from build123d import *

# Parameters (mm, degrees)
CROQUIS1_R              = 100
SALIENTE_EXTRUIR1_DEPTH = 3
CROQUIS3_R              = 110
CORTAR_EXTRUIR1_DEPTH   = 3
REDONDEO1_R             = 10
CROQUIS4_R              = 1.5
CROQUIS4_R_2            = 12.5
CORTAR_EXTRUIR2_DEPTH   = 142.453172607
CROQUIS5_R              = 1.5
CORTAR_EXTRUIR3_DEPTH   = 142.453172607
CROQUIS7_R              = 2
CORTAR_EXTRUIR5_DEPTH   = 10


with BuildPart() as part:
    # Croquis1 → Saliente-Extruir1 (new body)
    with BuildSketch(Plane.XY):
        Circle(CROQUIS1_R)
    extrude(amount=SALIENTE_EXTRUIR1_DEPTH)

    # Croquis3 → Cortar-Extruir1 (cut)
    with BuildSketch(Plane.XY.offset(3)):
        with Locations((190, 0)):
            Circle(CROQUIS3_R)
    extrude(amount=-CORTAR_EXTRUIR1_DEPTH, mode=Mode.SUBTRACT)

    # Redondeo1
    redondeo1_edges = [part.edges().sort_by_distance(p)[0] for p in [
        (89.473684211, -44.659375654, 1.5),
        (89.473684211, 44.659375654, 1.5),
    ]]
    fillet(redondeo1_edges, radius=REDONDEO1_R)

    # Croquis4 → Cortar-Extruir2 (cut, through all)
    with BuildSketch(Plane.XY.offset(3)):
        with Locations((-65.01846853, -38.219121523)):
            Circle(CROQUIS4_R)
        with Locations((-49.462119344, -22.662772337)):
            Circle(CROQUIS4_R)
        with Locations((-22.662772337, -49.462119344)):
            Circle(CROQUIS4_R)
        with Locations((-38.219121523, -65.01846853)):
            Circle(CROQUIS4_R)
        with Locations((-22.662772337, 49.462119344)):
            Circle(CROQUIS4_R)
        with Locations((-38.219121523, 65.01846853)):
            Circle(CROQUIS4_R)
        with Locations((-49.462119344, 22.662772337)):
            Circle(CROQUIS4_R)
        with Locations((-65.01846853, 38.219121523)):
            Circle(CROQUIS4_R)
        with Locations((49.462119344, 22.662772337)):
            Circle(CROQUIS4_R)
        with Locations((65.01846853, 38.219121523)):
            Circle(CROQUIS4_R)
        with Locations((22.662772337, 49.462119344)):
            Circle(CROQUIS4_R)
        with Locations((38.219121523, 65.01846853)):
            Circle(CROQUIS4_R)
        with Locations((22.662772337, -49.462119344)):
            Circle(CROQUIS4_R)
        with Locations((38.219121523, -65.01846853)):
            Circle(CROQUIS4_R)
        with Locations((49.462119344, -22.662772337)):
            Circle(CROQUIS4_R)
        with Locations((65.01846853, -38.219121523)):
            Circle(CROQUIS4_R)
        Circle(CROQUIS4_R_2)
        Polygon((-58.336309448, -83.085046789), (-83.085046789, -58.336309448), (-66.821590822, -42.072853481), (-42.072853481, -66.821590822), align=None)
        Polygon((-66.821590822, 42.072853481), (-42.072853481, 66.821590822), (-58.336309448, 83.085046789), (-83.085046789, 58.336309448), align=None)
        Polygon((42.072853481, 66.821590822), (66.821590822, 42.072853481), (83.085046789, 58.336309448), (58.336309448, 83.085046789), align=None)
        Polygon((66.821590822, -42.072853481), (42.072853481, -66.821590822), (58.336309448, -83.085046789), (83.085046789, -58.336309448), align=None)
    extrude(amount=-CORTAR_EXTRUIR2_DEPTH, mode=Mode.SUBTRACT)

    # Croquis5 → Cortar-Extruir3 (cut, through all)
    with BuildSketch(Plane(origin=(0, 0, 0), x_dir=(-1, 0, 0), z_dir=(0, 0, -1))):
        with Locations((11.5, -90)):
            Circle(CROQUIS5_R)
        with Locations((-11.5, -90)):
            Circle(CROQUIS5_R)
        with Locations((-11.5, -50)):
            Circle(CROQUIS5_R)
        with Locations((11.5, -50)):
            Circle(CROQUIS5_R)
        with Locations((-11.5, 90)):
            Circle(CROQUIS5_R)
        with Locations((11.5, 90)):
            Circle(CROQUIS5_R)
        with Locations((11.5, 50)):
            Circle(CROQUIS5_R)
        with Locations((-11.5, 50)):
            Circle(CROQUIS5_R)
    extrude(amount=-CORTAR_EXTRUIR3_DEPTH, mode=Mode.SUBTRACT)

    # Croquis7 → Cortar-Extruir5 (cut)
    with BuildSketch(Plane(origin=(0, 0, 0), x_dir=(-1, 0, 0), z_dir=(0, 0, -1))):
        with Locations((-27.065, -80.785)):
            Circle(CROQUIS7_R)
        with Locations((27.065, -80.785)):
            Circle(CROQUIS7_R)
        with Locations(Location((27.065, 80.785, 0), (0, 0, 180))):
            Circle(CROQUIS7_R)
        with Locations(Location((-27.065, 80.785, 0), (0, 0, 180))):
            Circle(CROQUIS7_R)
    extrude(amount=-CORTAR_EXTRUIR5_DEPTH, mode=Mode.SUBTRACT)


solid = part.part
Geometry: final body of the model. Coordinates: model frame, mm. A direction names the side the tool comes from. Round coordinates to 2 decimals unless told otherwise and drop trailing zeros. Loops run counter-clockwise (first coordinate to the right, second up) from the corner with the lowest first, then second, coordinate; pieces in that order, holes last. Notation, with made-up numbers: M 30,-15 L 87,-15 A15 cw 87,-8 Z; hole C 84,-17.5 d11. An arc over 180 degrees is marked long. Put each result on its own line as item: value. Start each with the question number.
(1) Set-up query: faces 5 (the face through (-74.514, 49.765, 1.521)), 6 (the face through (-49.55, 74.3, 1.52)), 7 (the face through (54.274, 54.62, 1.521)). Return all of +Z, -Z, +X, -X, +Y, -Y with unobstructed straight access to the full face (end or side cutting, diameter ignored); none if empty.
(2) Draft query along Y for faces 1 (the face through (11.923, 3.755, 1.521)), 2 (the face through (49.55, -74.3, 1.52)), 3 (the face through (-0.853, -99.996, 1.479)), 4 (the face through (0.853, 99.996, 1.479)). Return one class per face: +Y half, -Y half, draft (parallel to the pull), parting line (faces both ways), or undercut.
(3) Section query C-C (z = 1.5). State how many separate pieces and enclosed holes the cut face has, then the cut area to 3 significant figures.
(4) Material intervals for line 1 along Y through (x, z) = (0, 0.85); line 2 along Y through (x, z) = (-22, 1.3); line 3 along Y through (x, z) = (11.5, 1.7), sorted ascending. Write a range as [from, to].
(5) Section query A-A (y = 72.5). Return loops of the section in (x, z), then the cut area to 3 significant figures.
(6) Section query B-B (x = -86). Return loops of the section in (y, z).
(7) Contact query for flat-ended pins moving along their axis: pin 1 Ø4.5 at (x, y) = (27.065, 80.785) entering from +Z; pin 2 Ø1.8 at (x, y) = (-22.66, -49.46) entering from +Z. Output: stop coordinate, or through.
Findings below:
1. face 5: +Z, -Z, +Y
1. face 6: +Z, -Z, -X
1. face 7: +Z, -Z
2. face 1: undercut
2. face 2: undercut
2. face 3: -Y half
2. face 4: +Y half
3. separate pieces: 1
3. enclosed holes: 29
3. area: 26,300 mm2
4. line 1: y = [-100, -12.5], [12.5, 100]
4. line 2: y = [-97.55, -50.81], [-48.12, 48.12], [50.81, 97.55]
4. line 3: y = [-99.34, -91.5], [-88.5, -51.5], [-48.5, -4.9], [4.9, 48.5], [51.5, 88.5], [91.5, 99.34]
5. outline: M -47.75,0 L 47.75,0 L 47.75,3 L -47.75,3 Z
5. area: 287 mm2
6. outline: M -51.03,0 L 51.03,0 L 51.03,3 L -51.03,3 Z
7. pin 1: stops at z = 3
7. pin 2: passes through
